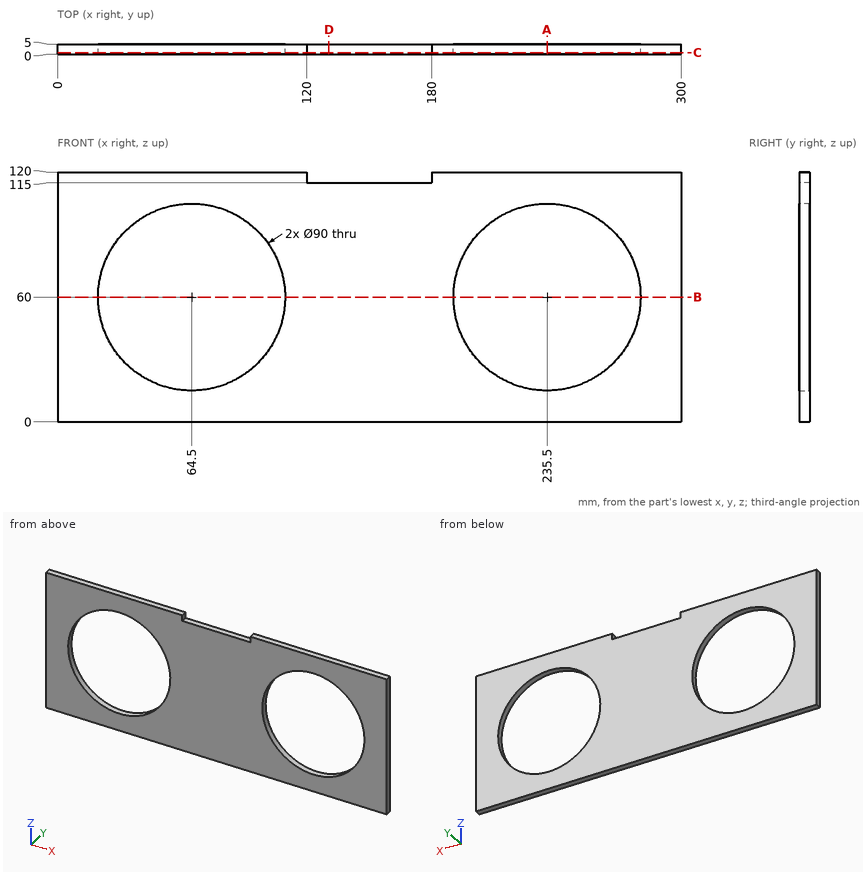
Answer from the drawing. Dimensions are ordinates in mm from the lowest x, y and z of the part. Coordinates: 2 decimals unless noted, no trailing zeros. Write each loop counter-clockwise with the first axis right and the second up, starting at its lowest first coordinate (ties: lowest second). Pieces come first, ordered by that corner, then holes. Notation, with made-up numbers: M 28.25,-17 L 53.25,-17 A15 cw 53.25,-4 Z; hole C -15,-22 d11. An arc over 180 degrees is marked long. Use one line per item in the form item = value. Start each with the question number.
1. Straight lines are drawn through the part: probe 1 along X at (y, z) = (1.4, 60); probe 2 along X at (y, z) = (2.75, 46); probe 3 along Z at (x, y) = (123, 2.3). For each, find the intervals that lie inside material, in ascending order. Write a range as from..to.
2. The part is cut by section D-D (x = 130.5). Give the vertices of the cut face in (y, z), plus the area to 3 significant figures.
3. The part is cut by section A-A (x = 235.5). Give the vertices of the cut face in (y, z), plus the area to 3 significant figures.
4. The part is cut by section C-C (y = 0.8). Give the vertices of the cut face in (x, z).
5. The part is cut by section B-B (z = 60). Give the vertices of the cut face in (x, y).
Evaluation:
q1.probe_1 = 0..19.5, 109.5..190.5, 280.5..300
q1.probe_2 = 0..21.73, 107.27..192.73, 278.27..300
q1.probe_3 = 0..115
q2.outline = M 0,0 L 5,0 L 5,115 L 0,115 Z
q2.area = 575 mm^2
q3.outline = M 0,0 L 5,0 L 5,15 L 0,15 Z; M 0,105 L 5,105 L 5,120 L 0,120 Z
q3.area = 150 mm^2
q4.outline = M 0,0 L 300,0 L 300,120 L 180,120 L 180,115 L 120,115 L 120,120 L 0,120 Z; hole C 64.5,60 d90; hole C 235.5,60 d90
q5.outline = M 0,0 L 19.5,0 L 19.5,5 L 0,5 Z; M 109.5,0 L 190.5,0 L 190.5,5 L 109.5,5 Z; M 280.5,0 L 300,0 L 300,5 L 280.5,5 Z
